Could you check a few things on this model? Use its own coordinates, in mm. Face numbers are marked on the shaded views. A direction names the side the tool comes from. Coordinates: 2 decimals unless noted, no trailing zeros. Loops run counter-clockwise (first coordinate to the right, second up) from the corner with the lowest first, then second, coordinate; pieces in that order, holes last. Notation, with made-up numbers: (49.25, 3.25) - (66.25, 3.25) arc R16 ccw to (66.25, 18.25) - close; hole circle Ø7 at (87, 9). An arc over 180 degrees is marked (long way). One line per item, written item: value. Start each with the question number.
(1) On a 3-axis mill with a long thin cutter (end or side, diameter ignored), from which of +Z, -Z, +X, -X, +Y, -Y can I reach the whole of each face in a straight line? I mean the marked faces 1, 2, 3, 4 and 5. Say none if no direction works.
(2) If we section it at D-D on y = -9: Write out the boundary of the cut face in (x, z).
(3) I'm going to push flat-ended pins straight in: P1, Ø2.5, axis at y = -2.5, z = 6.5, coming from the -X side; P2, Ø5, axis at x = 20.5, z = 5.5, coming from the -Y side; P3, Ø5, axis at y = -3, z = 8, coming from the -X side; P4, Ø5, axis at x = 24.5, z = 6.5, coming from the +Y side. Where does each tip first touch, or does it pass through?
(4) If we section it at A-A on z = 2.5: Write out the boundary of the cut face in (x, y), then the cut area to 3 significant figures.
(5) If we section it at B-B on z = 9.25: Write out the boundary of the cut face in (x, y).
(6) If I drill on line 1 along X through (y, z) = (0.5, 4.25); line 2 along Y through (x, z) = (4, 3.25); line 3 along X through (y, z) = (-27, 4), over which ranges is the centre line in solid material (lowest first)? Write a range as from..to.
(7) If we mould it in two halves opening along X, with no side actions, what happens to the marked faces 6, 7 and 8? For each: pulls with the +X half, pulls with the -X half, needs draft (parallel to the pull), parting line crosses it, or undercut.
(8) If we section it at C-C on x = 14: Write out the boundary of the cut face in (y, z).
```python
from build123d import *

# Parameters (mm, degrees)
F0_W     = 4.8
F0_H     = 10
F0_W_2   = 10
F0_H_2   = 4.95
F0_H_3   = 4.85
F0_W_3   = 4.9
F1_DEPTH = 10
F3_DEPTH = 5


with BuildPart() as f1:
    # F0 (on Top) → F1 (new body)
    with BuildSketch(Plane.XY):
        Polygon((5.2, 0), (0, 0), (0, -5.05), (0, -10), (0, -14.95), (0, -20), (5.1, -20), (10, -20), (14.9, -20), (20, -20), (20, -14.85), (20, -10), (20, -5.15), (20, 0), (14.8, 0), (10, 0), align=None)
        with Locations((7.6, 5)):
            Rectangle(F0_W, F0_H)
        with Locations((-5, -7.525)):
            Rectangle(F0_W_2, F0_H_2)
        with Locations((12.4, 5)):
            Rectangle(F0_W, F0_H)
        with Locations((-5, -12.475)):
            Rectangle(F0_W_2, F0_H_2)
        with Locations((25, -7.575)):
            Rectangle(F0_W_2, F0_H_3)
        with Locations((7.55, -25)):
            Rectangle(F0_W_3, F0_H)
        with Locations((25, -12.425)):
            Rectangle(F0_W_2, F0_H_3)
        with Locations((12.45, -25)):
            Rectangle(F0_W_3, F0_H)
    extrude(amount=F1_DEPTH)

    # F2 (on face) → F3 (cut)
    with BuildSketch(Plane.XY.offset(10)):
        Polygon((10, -14.9), (15.18014, -14.874099), (9.949831, -4.866128), align=None)
        Polygon((4.301277, -14.928494), (10, -14.9), (9.949831, -4.866128), align=None)
    extrude(amount=-F3_DEPTH, mode=Mode.SUBTRACT)


solid = f1.part
```
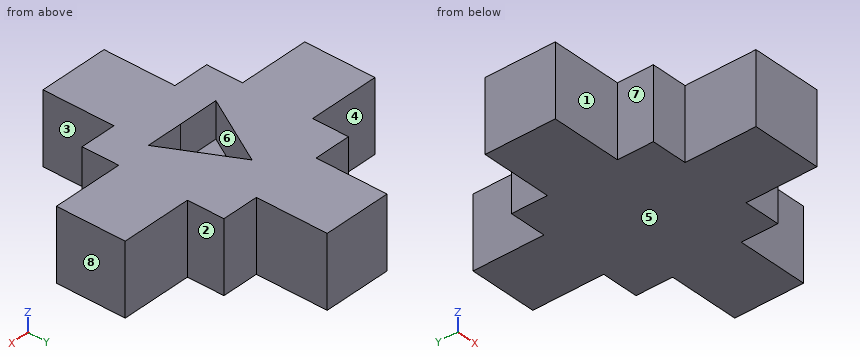
Values:
1. face 1: +Z, -Z, -X, -Y
1. face 2: +Z, -Z, +X, +Y
1. face 3: +Z, -Z, +X, -Y
1. face 4: +Z, -Z, -X, +Y
1. face 5: -Z, +X, -X, +Y, -Y
2. outline: (-10, 0) - (30, 0) - (30, 10) - (12.11, 10) - (12.11, 5) - (7.63, 5) - (7.63, 10) - (-10, 10) - close
3. P1: stops at x = 0
3. P2: stops at y = -20
3. P3: stops at x = -10
3. P4: stops at y = -5.15
4. outline: (-10, -14.95) - (0, -14.95) - (0, -20) - (5.1, -20) - (5.1, -30) - (14.9, -30) - (14.9, -20) - (20, -20) - (20, -14.85) - (30, -14.85) - (30, -5.15) - (20, -5.15) - (20, 0) - (14.8, 0) - (14.8, 10) - (5.2, 10) - (5.2, 0) - (0, 0) - (0, -5.05) - (-10, -5.05) - close
4. area: 790 mm2
5. outline: (-10, -14.95) - (0, -14.95) - (0, -20) - (5.1, -20) - (5.1, -30) - (14.9, -30) - (14.9, -20) - (20, -20) - (20, -14.85) - (30, -14.85) - (30, -5.15) - (20, -5.15) - (20, 0) - (14.8, 0) - (14.8, 10) - (5.2, 10) - (5.2, 0) - (0, 0) - (0, -5.05) - (-10, -5.05) - close; hole (4.3, -14.93) - (15.18, -14.87) - (9.95, -4.87) - close
6. line 1: x = 5.2..14.8
6. line 2: y = -20..0
6. line 3: x = 5.1..14.9
7. face 6: undercut
7. face 7: pulls with the -X half
7. face 8: pulls with the +X half
8. outline: (-30, 0) - (10, 0) - (10, 10) - (-12.62, 10) - (-12.62, 5) - (-14.88, 5) - (-14.88, 10) - (-30, 10) - close
